For this review, take the finished solid that the model builds, in its own axes (mm). Face numbers are marked on the shaded views. A direction names the side the tool comes from. Round coordinates to 2 decimals unless told otherwise and drop trailing zeros. Loops run counter-clockwise (first coordinate to the right, second up) from the corner with the lowest first, then second, coordinate; pieces in that order, holes last.
1. Consider section A-A on x = 0. State the section outline as (y, z) points, then the cut area to 3 significant figures.
2. Tool access review of the marked faces 4 and 5: name each direction out of +Z, -Z, +X, -X, +Y, -Y from which nothing blocks a thin tool from reaching the whole face with its end or side.
3. Clearance check with flat-ended pins moving along their axes: pin 1 Ø6 at (x, y) = (0.5, 2.5) entering from +Z; pin 2 Ø1 at (y, z) = (6, 8.5) entering from -X; pin 3 Ø1.5 at (x, z) = (-7.5, 20.5) entering from +Y. State where each tip first meets the part, or that it passes through.
4. Draft analysis for pull direction X (two halves, no side actions). For the marked faces 1, 2 and 3, state which applies: released by +X, released by -X, zero draft, split by the parting line, or undercut.
5. To check wall thickness, follow line 1 along Z through (x, y) = (-4.75, 1); line 2 along Z through (x, y) = (5.25, 5); line 3 along Y through (x, z) = (-8.25, 14). State the ranges of each line that lie inside material, in increasing order.
6. Consider section B-B on z = 35. State the section outline as (x, y) points, then the cut area to 3 significant figures.
from build123d import *

# Parameters (mm, degrees)
SKETCH1_R           = 10.5
BOSS_EXTRUDE1_DEPTH = 40.5
SHELL1_T            = -4
FILLET1_R           = 3.5
FILLET2_R           = 3.5
FILLET3_R           = 1
SKETCH2_W           = 37.590072207
SKETCH2_H           = 54.748834579
CUT_EXTRUDE1_DEPTH  = 40.5


with BuildPart() as part:
    # Sketch1 → Boss-Extrude1 (new body)
    with BuildSketch(Plane.XY):
        Circle(SKETCH1_R)
    extrude(amount=BOSS_EXTRUDE1_DEPTH)

    # Shell1
    shell1_openings = [part.faces().sort_by_distance(p)[0] for p in [
        (0, 0, 40.5),
    ]]
    offset(amount=SHELL1_T, openings=shell1_openings, kind=Kind.INTERSECTION)

    # Fillet1
    fillet1_edges = [part.edges().sort_by_distance(p)[0] for p in [
        (-10.5, 0, 40.5),
    ]]
    fillet(fillet1_edges, radius=FILLET1_R)

    # Fillet2
    fillet2_edges = [part.edges().sort_by_distance(p)[0] for p in [
        (-10.5, 0, 0),
    ]]
    fillet(fillet2_edges, radius=FILLET2_R)

    # Fillet3
    fillet3_edges = [part.edges().sort_by_distance(p)[0] for p in [
        (-6.5, 0, 4),
    ]]
    fillet(fillet3_edges, radius=FILLET3_R)

    # Sketch2 → Cut-Extrude1 (cut)
    with BuildSketch(Plane(origin=(0, 0, 0), x_dir=(1, 0, 0), z_dir=(0, 1, 0))):
        with Locations((0.840248673, -18.259937353)):
            Rectangle(SKETCH2_W, SKETCH2_H)
    extrude(amount=-CUT_EXTRUDE1_DEPTH, mode=Mode.SUBTRACT)


solid = part.part
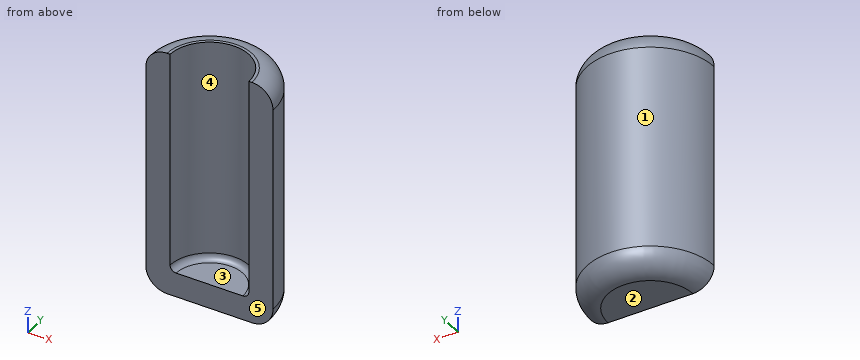
Resolved:
1. outline: (0, 0) - (7, 0) arc R3.5 ccw to (10.5, 3.5) - (10.5, 37) arc R3.5 ccw to (7, 40.5) - (6.5, 40.5) - (6.5, 5) arc R1 cw to (5.5, 4) - (0, 4) - close
1. area: 183 mm2
2. face 4: +Z, -Y
2. face 5: +Z, -Z, +X, -X, -Y
3. pin 1: stops at z = 4
3. pin 2: stops at x = -8.94
3. pin 3: stops at y = 8.04
4. face 1: split by the parting line
4. face 2: zero draft
4. face 3: undercut
5. line 1: z = 0 to 4
5. line 2: z = 0.01 to 40.49
5. line 3: y = 0 to 6.5
6. outline: (-10.5, 0) - (-6.5, 0) arc R6.5 cw to (6.5, 0) - (10.5, 0) arc R10.5 ccw to start
6. area: 107 mm2
